from build123d import *

# Parameters (mm, degrees)
SKETCH_1_R          = 2
SKETCH_1_W          = 3
SKETCH_1_H          = 8
SKETCH_1_W_2        = 8
SKETCH_1_H_2        = 3
EXTRUDE_1_DEPTH     = 3
SKETCH_2_R          = 4
CUT_EXTRUDE_1_DEPTH = 10
SKETCH_3_W          = 70
SKETCH_3_H          = 15
CUT_EXTRUDE_2_DEPTH = 10
SKETCH_4_W          = 20
SKETCH_4_H          = 40
CUT_EXTRUDE_3_DEPTH = 10
FILLET_1_R          = 3
FILLET_2_R          = 6


with BuildPart() as part:
    # 草图1 → 凸台-拉伸1 (new body)
    with BuildSketch(Plane(origin=(0, 0, 0), x_dir=(1, 0, 0), z_dir=(0, 1, 0))):
        Polygon((-35, -45), (-10, -85), (10, -85), (35, -45), (35, 45), (-35, 45), align=None)
        with Locations(Location((0, -55, 0), (0, 0, 270))):
            Circle(SKETCH_1_R, mode=Mode.SUBTRACT)
        with Locations(Location((0, -75, 0), (0, 0, 270))):
            Circle(SKETCH_1_R, mode=Mode.SUBTRACT)
        with Locations((-24, 13.5)):
            Rectangle(SKETCH_1_W, SKETCH_1_H, mode=Mode.SUBTRACT)
        with Locations((-24, -13.5)):
            Rectangle(SKETCH_1_W, SKETCH_1_H, mode=Mode.SUBTRACT)
        with Locations((13.5, 24)):
            Rectangle(SKETCH_1_W_2, SKETCH_1_H_2, mode=Mode.SUBTRACT)
        with Locations((-13.5, 24)):
            Rectangle(SKETCH_1_W_2, SKETCH_1_H_2, mode=Mode.SUBTRACT)
        with Locations((-13.5, -24)):
            Rectangle(SKETCH_1_W_2, SKETCH_1_H_2, mode=Mode.SUBTRACT)
        with Locations((13.5, -24)):
            Rectangle(SKETCH_1_W_2, SKETCH_1_H_2, mode=Mode.SUBTRACT)
        with Locations((24, 13.5)):
            Rectangle(SKETCH_1_W, SKETCH_1_H, mode=Mode.SUBTRACT)
        with Locations((24, -13.5)):
            Rectangle(SKETCH_1_W, SKETCH_1_H, mode=Mode.SUBTRACT)
    extrude(amount=EXTRUDE_1_DEPTH)

    # 草图2 → 切除-拉伸1 (cut)
    with BuildSketch(Plane(origin=(0, 3, 0), x_dir=(1, 0, 0), z_dir=(0, 1, 0))):
        with Locations(Location((0, -35, 0), (0, 0, 270))):
            Circle(SKETCH_2_R)
        with Locations(Location((-20, -35, 0), (0, 0, 270))):
            Circle(SKETCH_2_R)
        with Locations(Location((20, -35, 0), (0, 0, 270))):
            Circle(SKETCH_2_R)
    extrude(amount=-CUT_EXTRUDE_1_DEPTH, mode=Mode.SUBTRACT)

    # 草图3 → 切除-拉伸2 (cut)
    with BuildSketch(Plane(origin=(0, 3, 0), x_dir=(1, 0, 0), z_dir=(0, 1, 0))):
        with Locations((0, 37.5)):
            Rectangle(SKETCH_3_W, SKETCH_3_H)
    extrude(amount=-CUT_EXTRUDE_2_DEPTH, mode=Mode.SUBTRACT)

    # 草图4 → 切除-拉伸3 (cut)
    with BuildSketch(Plane(origin=(0, 3, 0), x_dir=(1, 0, 0), z_dir=(0, 1, 0))):
        Rectangle(SKETCH_4_W, SKETCH_4_H)
    extrude(amount=-CUT_EXTRUDE_3_DEPTH, mode=Mode.SUBTRACT)

    # 圆角1
    fillet_1_edges = [part.edges().sort_by_distance(p)[0] for p in [
        (10, 1.5, -20),
        (10, 1.5, 20),
        (-10, 1.5, 20),
        (-10, 1.5, -20),
    ]]
    fillet(fillet_1_edges, radius=FILLET_1_R)

    # 圆角2
    fillet_2_edges = [part.edges().sort_by_distance(p)[0] for p in [
        (-35, 1.5, -30),
        (35, 1.5, -30),
        (-10, 1.5, 85),
        (-35, 1.5, 45),
        (35, 1.5, 45),
        (10, 1.5, 85),
    ]]
    fillet(fillet_2_edges, radius=FILLET_2_R)


solid = part.part
CAD build for the part. Positions are in the model's coordinates, mm. Coordinates: 2 decimals unless noted, no trailing zeros. Write each loop counter-clockwise with the first axis right and the second up, starting at its lowest first coordinate (ties: lowest second). Pieces come first, ordered by that corner, then holes. Notation, with made-up numbers: M 41.5,-30.75 L 80.5,-30.75 A22 ccw 80.5,-5.75 Z; hole C 30.5,-6.5 d5. An arc over 180 degrees is marked long. Return JSON: item names as keys, results as strings.
Item 1: Slice it at A-A, the plane z = -3. Write the cut outline in (x, y).
Findings below:
{"outline": "M -35,0 L -10,0 L -10,3 L -35,3 Z; M 10,0 L 35,0 L 35,3 L 10,3 Z"}
Item 2: Slice it at D-D, the plane x = 20. Write the cut outline in (y, z).
Findings below:
{"outline": "M 0,-30 L 3,-30 L 3,31 L 0,31 Z; M 0,39 L 3,39 L 3,69 L 0,69 Z"}
Item 3: Slice it at B-B, the plane z = 35. Write the cut outline in (x, y).
Findings below:
{"outline": "M -35,0 L -24,0 L -24,3 L -35,3 Z; M -16,0 L -4,0 L -4,3 L -16,3 Z; M 4,0 L 16,0 L 16,3 L 4,3 Z; M 24,0 L 35,0 L 35,3 L 24,3 Z"}
Item 4: Slice it at C-C, the plane x = 0. Write the cut outline in (y, z).
Findings below:
{"outline": "M 0,-30 L 3,-30 L 3,-20 L 0,-20 Z; M 0,20 L 3,20 L 3,31 L 0,31 Z; M 0,39 L 3,39 L 3,53 L 0,53 Z; M 0,57 L 3,57 L 3,73 L 0,73 Z; M 0,77 L 3,77 L 3,85 L 0,85 Z"}
Item 5: Drop flat-ended pins along their axis: pin 1 Ø0.9 at (x, y) = (24, 2) entering from +Z; pin 2 Ø1.5 at (x, y) = (-12.5, 1.5) entering from +Z; pin 3 Ø1.5 at (x, y) = (-23.5, 1) entering from +Z. Give the stop position or say it passes through.
Findings below:
{"pin 1": "stops at z = 63.32", "pin 2": "stops at z = 82.2", "pin 3": "stops at z = 64.6"}
Item 6: Two-plate mould, pull along Z, no slides. Class faces 1 (the flat face through (0, 0, 27)), 2 (the cylindrical face through (-33.289, 1.479, -28.196)), 3 (the flat face through (0, 1, 85)), 4 (the flat face through (-14, 1, 25.5)): +Z half, -Z half, draft (parallel to the pull), parting line (faces both ways), or undercut.
Findings below:
{"face 1": "draft", "face 2": "-Z half", "face 3": "+Z half", "face 4": "undercut"}
Item 7: Probe line 1 (X direction, y = 1.5, z = 23); line 2 (X direction, y = 1.2, z = 35); line 3 (Z direction, x = 3, y = 2.1). List the from-to ranges inside material, lowest first. Write a range as from..to.
Findings below:
{"line 1": "x = -35..-17.5, -9.5..9.5, 17.5..35", "line 2": "x = -35..-24, -16..-4, 4..16, 24..35", "line 3": "z = -30..-20, 20..32.35, 37.65..85"}
